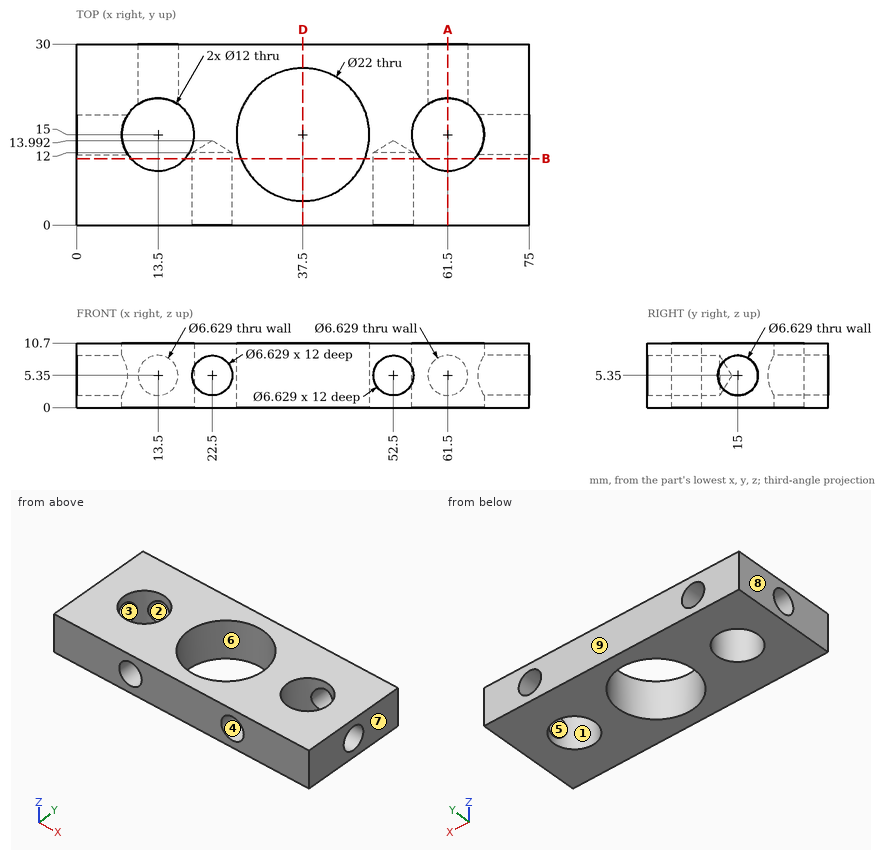
Geometry check sheet. Reference: drawing and pictorial views, mm from the part's lowest x, y, z. A direction names the side the tool comes from. Round coordinates to 2 decimals unless told otherwise and drop trailing zeros. Loops run counter-clockwise (first coordinate to the right, second up) from the corner with the lowest first, then second, coordinate; pieces in that order, holes last.
1. Gauge pin test, flat ends, axial feed: pin 1 Ø6 at (x, z) = (52.5, 5.35) entering from -Y; pin 2 Ø4 at (x, z) = (61.5, 5.35) entering from +Y; pin 3 Ø4 at (y, z) = (15, 5.35) entering from +X. Record the tip position at first contact, or that the pin passes through.
2. Mould release check, pull along X, two halves, no side actions. Record for the marked faces 6, 7, 8 and 9: released by +X, released by -X, zero draft, split by the parting line, or undercut.
3. Scan lines: probe 1 along Z at (x, y) = (13.5, 27.5) (1 decimal); probe 2 along Y at (x, z) = (38, 2.75); probe 3 along X at (y, z) = (3.5, 8.25) (1 decimal). Record each from-to range of solid material in increasing order.
4. Sectioned sample at D-D on x = 37.5. Record the boundary of the cut face in (y, z), and give its area (3 significant figures).
5. Set-up check for the marked faces 1, 2, 3, 4 and 5: record each of +Z, -Z, +X, -X, +Y, -Y from which the full face is reachable in a straight line by a thin tool's end or side.
6. Sectioned sample at A-A on x = 61.5. Record the boundary of the cut face in (y, z) (1 decimal), and give its area (3 significant figures).
7. Sectioned sample at B-B on y = 11. Give the number of separate pieces and of enclosed holes in the cut face, and give its area (3 significant figures).
Recorded:
1. pin 1: stops at y = 12.19
1. pin 2: stops at y = 9.34
1. pin 3: stops at x = 55.84
2. face 6: undercut
2. face 7: released by +X
2. face 8: released by -X
2. face 9: zero draft
3. probe 1: z = 0 to 2, 8.7 to 10.7
3. probe 2: y = 0 to 4.01, 25.99 to 30
3. probe 3: x = 0 to 20.9, 24.1 to 50.9, 54.1 to 75
4. outline: (0, 0) - (4, 0) - (4, 10.7) - (0, 10.7) - close; (26, 0) - (30, 0) - (30, 10.7) - (26, 10.7) - close
4. area: 85.6 mm2
5. face 1: +Z, -Z
5. face 2: +Y
5. face 3: -X
5. face 4: -Y
5. face 5: +X
6. outline: (0, 0) - (9, 0) - (9, 10.7) - (0, 10.7) - close; (21, 0) - (30, 0) - (30, 2) - (21, 2) - close; (21, 8.7) - (30, 8.7) - (30, 10.7) - (21, 10.7) - close
6. area: 133 mm2
7. separate pieces: 4
7. enclosed holes: 2
7. area: 323 mm2
